For this review, take the finished solid that the model builds, in its own axes (mm). Give positions to 0.01 mm unless a question says otherwise; leave off trailing zeros. Order: outer loops, then holes, each group sorted by start corner. A loop starts at its lowest first (then second) coordinate and runs counter-clockwise, first axis right, second up. Notation, with made-up numbers: (25.25, 22) - (71.25, 22) arc R25 ccw to (71.25, 59) - close; hole circle Ø4 at (46, 7). An arc over 180 degrees is marked (long way). Use a Markdown table: item, result. Add a question column.
1) We need section A-A on x = 0. Write out the cut boundary in (y, z), then the cut area to 3 significant figures.
2) Wall thickness on L1, parallel to Y at x = 0, z = 2.65; L2, parallel to Z at x = 5.5, y = -0.25; L3, parallel to Y at x = -1.75, z = 1.65 (3 decimals): over which ranges is each line inside the solid? List them lowest first.
3) Mouldability with a two-part tool opening along Y and no side actions: class faces 1 (the face through (3, -7, 1.9)), 2 (the face through (1.96, -1.81, 2.28)), 3 (the face through (-4.4, -5.3, 2.6)) as released by +Y, released by -Y, zero draft, split by the parting line, or undercut.
4) We need section B-B on z = 1.05. Write out the cut boundary in (x, y), then the cut area to 3 significant figures.
5) Clearance check with a flat-ended pin moving along its axis: P1, Ø1, axis at x = -6, y = -0.5, coming from the +Z side. State where the tip first meets the part, or that it passes through.
```python
from build123d import *

# Parameters (mm, degrees)
F0_R     = 5.5
F0_R_2   = 2
F1_DEPTH = 3.3
F0_R_3   = 8
F2_DEPTH = 1.9
F3_SIZE  = 2.4
F4_SIZE  = 0.3


# Not quite as in the source:
# - a feature names something its author has since deleted; it is built from what else it names


with BuildPart() as f1:
    # F0 (on Top) → F1 (new body)
    with BuildSketch(Plane.XY):
        with Locations((0, -2)):
            Circle(F0_R)
        with Locations((0, -0.9976860601)):
            Circle(F0_R_2, mode=Mode.SUBTRACT)
    extrude(amount=F1_DEPTH)

    # F0 (on Top) → F2 (join)
    with BuildSketch(Plane.XY):
        with Locations((0, -2)):
            Circle(F0_R_3)
        with Locations((0, -2)):
            Circle(F0_R, mode=Mode.SUBTRACT)
    extrude(amount=F2_DEPTH)

    # F3
    f3_edges = [f1.edges().sort_by_distance(p)[0] for p in [
        (-2, -0.997686, 0),
    ]]
    chamfer(f3_edges, length=F3_SIZE)

    # F4
    f4_edges = [f1.edges().sort_by_distance(p)[0] for p in [
        (-8, -2, 1.9),
        (-8, -2, 0),
    ]]
    chamfer(f4_edges, length=F4_SIZE)


solid = f1.part
```
Checked values:
| question | item | result |
|---|---|---|
| 1 | outline | (-10, 0.3) - (-9.7, 0) - (-5.4, 0) - (-3, 2.4) - (-3, 3.3) - (-7.5, 3.3) - (-7.5, 1.9) - (-9.7, 1.9) - (-10, 1.6) - close; (1, 2.4) - (3.4, 0) - (5.7, 0) - (6, 0.3) - (6, 1.6) - (5.7, 1.9) - (3.5, 1.9) - (3.5, 3.3) - (1, 3.3) - close |
| 1 | area | 26.7 mm² |
| 2 | L1 | -7.5 to -3, 1 to 3.5 |
| 2 | L2 | 0 to 1.9 |
| 2 | L3 | -9.755 to -3.119, 1.124 to 5.755 |
| 3 | face 1 | zero draft |
| 3 | face 2 | undercut |
| 3 | face 3 | split by the parting line |
| 4 | outline | circle Ø16 at (0, -2); hole circle Ø6.7 at (0, -1) |
| 4 | area | 166 mm² |
| 5 | P1 | z = 1.9 |
